Input: part model. Units: mm. Frame: model coordinates. A direction names the side the tool comes from. Coordinates: 2 decimals unless noted, no trailing zeros. Loops run counter-clockwise (first coordinate to the right, second up) from the corner with the lowest first, then second, coordinate; pieces in that order, holes last. Notation, with made-up numbers: (6.25, -29) - (47.25, -29) arc R32 cw to (47.25, 0) - close; hole circle Ø7 at (21, -24). An arc over 180 degrees is marked (long way). Use one line per item in the form item = value.
from build123d import *

# Parameters (mm, degrees)
F_6_32_TAPPED_HOLE1_D = 2.7051
CIRPATTERN1_COUNT     = 8


with BuildPart() as part:
    # Sketch1 → Revolve1 (revolve)
    with BuildSketch(Plane.XY, mode=Mode.PRIVATE) as revolve1_sk:
        Polygon((-12.7, 4.7625), (-12.7, 0.79375), (-1.190625, 0.79375), (-1.190625, 2.778125), (-6.35, 2.778125), (-6.35, 4.7625), align=None)
    revolve(revolve1_sk.sketch.rotate(Axis((0, 0, 0), (0, 1, 0)), 270), axis=Axis((0, 0, 0), (0, 1, 0)))

    # #6-32 Tapped Hole1 (through all)
    with Locations(Plane(origin=(0, 4.7625, 0), x_dir=(1, 0, 0), z_dir=(0, 1, 0))):
        with Locations((9.779, 0)):
            f_6_32_tapped_hole1 = Hole(F_6_32_TAPPED_HOLE1_D / 2)

    # CirPattern1: #6-32 Tapped Hole1 ×8 about axis
    cirpattern1_axis = Axis((0, 0, 0), (0, 1, 0))
    for i in range(1, CIRPATTERN1_COUNT):
        add(f_6_32_tapped_hole1.rotate(cirpattern1_axis, i * 360 / CIRPATTERN1_COUNT), mode=Mode.SUBTRACT)


solid = part.part
Q1. First-contact query: P1, Ø1.6, axis at x = 0, z = -9.779, coming from the +Y side; P2, Ø4, axis at x = 0, z = 0, coming from the +Y side; P3, Ø2, axis at y = 2, z = -1.5, coming from the +X side. Flat tips, straight axial feed; report the tip coordinate or a pass-through.
Check values:
P1 = through
P2 = 2.78
P3 = 12.69
Q2. Set-up query: faces 5 (the cylindrical face through (0.06, 2.75, 11.13)), 6 (the cylindrical face through (3.86, 3.78, 5.04)). Return all of +Z, -Z, +X, -X, +Y, -Y with unobstructed straight access to the full face (end or side cutting, diameter ignored); none if empty.
Check values:
face_5 = +Y, -Y
face_6 = +Y
Q3. Cut plane D-D, the plane x = -10.5. Return loops of the section in (y, z), then the cut area to 3 significant figures.
Check values:
outline = (0.79, -7.14) - (4.76, -7.14) - (4.76, -1.14) - (0.79, -1.14) - close; (0.79, 1.14) - (4.76, 1.14) - (4.76, 7.14) - (0.79, 7.14) - close
area = 47.6 mm²
Q4. Cut plane A-A, the plane x = 0. Return loops of the section in (y, z).
Check values:
outline = (0.79, -12.7) - (4.76, -12.7) - (4.76, -11.13) - (0.79, -11.13) - close; (0.79, -8.43) - (4.76, -8.43) - (4.76, -6.35) - (2.78, -6.35) - (2.78, -1.19) - (0.79, -1.19) - close; (0.79, 1.19) - (2.78, 1.19) - (2.78, 6.35) - (4.76, 6.35) - (4.76, 8.43) - (0.79, 8.43) - close; (0.79, 11.13) - (4.76, 11.13) - (4.76, 12.7) - (0.79, 12.7) - close
Q5. Cut plane C-C, the plane z = 9. Return loops of the section in (x, y).
Check values:
outline = (-8.96, 0.79) - (-1.11, 0.79) - (-1.11, 4.76) - (-8.96, 4.76) - close; (1.11, 0.79) - (8.96, 0.79) - (8.96, 4.76) - (1.11, 4.76) - close
Q6. Pull-direction query (X, two-part tool) for faces 1 (the cylindrical face through (11.13, 2.75, -0.06)), 2 (the cylindrical face through (7.83, 2.75, -7.91)), 3 (the cylindrical face through (7.7, 2.8, 10.1)), 4 (the flat face through (-6, 4.762, 3)); classes: pulls with the +X half, pulls with the -X half, needs draft (parallel to the pull), parting line crosses it, or undercut.
Check values:
face_1 = undercut
face_2 = undercut
face_3 = parting line crosses it
face_4 = needs draft
Q7. Ray query, line 1 along X through (y, z) = (3.65, 6.5); line 2 along Z through (x, y) = (-6.25, 1.5); line 3 along Z through (x, y) = (6.75, 2.4). Return the intervals inside material, ascending. Write a range as [from, to].
Check values:
line_1 = [-10.91, -8.2], [-5.63, 5.63], [8.2, 10.91]
line_2 = [-11.06, -8.09], [-5.74, 5.74], [8.09, 11.06]
line_3 = [-10.76, -8.26], [-5.57, 5.57], [8.26, 10.76]
Q8. Cut plane B-B, the plane z = 0. Return loops of the section in (x, y), then the cut area to 3 significant figures.
Check values:
outline = (-12.7, 0.79) - (-11.13, 0.79) - (-11.13, 4.76) - (-12.7, 4.76) - close; (-8.43, 0.79) - (-1.19, 0.79) - (-1.19, 2.78) - (-6.35, 2.78) - (-6.35, 4.76) - (-8.43, 4.76) - close; (1.19, 0.79) - (8.43, 0.79) - (8.43, 4.76) - (6.35, 4.76) - (6.35, 2.78) - (1.19, 2.78) - close; (11.13, 0.79) - (12.7, 0.79) - (12.7, 4.76) - (11.13, 4.76) - close
area = 49.4 mm²
